from build123d import *

# Parameters (mm, degrees)
SALIENTE_EXTRUIR1_DEPTH = 4
SALIENTE_EXTRUIR2_DEPTH = 6.2
CORTAR_EXTRUIR1_REACH   = 20.8
CROQUIS3_R              = 1.6
CORTAR_EXTRUIR2_DEPTH   = 3
SALIENTE_EXTRUIR3_DEPTH = 8.4
SALIENTE_EXTRUIR4_DEPTH = 10


with BuildPart() as part:
    # Croquis1 → Saliente-Extruir1 (new body)
    with BuildSketch(Plane.XY):
        Polygon((0, 0), (25, 0), (25, 5), (13.5, 5), (13.5, 35), (0, 35), align=None)
    extrude(amount=SALIENTE_EXTRUIR1_DEPTH)

    # Croquis2 → Saliente-Extruir2 (add)
    with BuildSketch(Plane.XY.offset(4)):
        Polygon((6.2, 35), (6.2, 0), (25, 0), (25, 5), (13.5, 5), (13.5, 35), align=None)
    extrude(amount=SALIENTE_EXTRUIR2_DEPTH)

    # Croquis3 → Cortar-Extruir1 (cut, up to next)
    with BuildSketch(Plane.ZY.offset(-6.2), mode=Mode.PRIVATE) as cortar_extruir1_sk1:
        with Locations((7.1, 24.3)):
            Circle(CROQUIS3_R)
    cortar_extruir1_tool1 = extrude(cortar_extruir1_sk1.sketch, amount=-CORTAR_EXTRUIR1_REACH, mode=Mode.PRIVATE) & part.part
    add(cortar_extruir1_tool1.solids().sort_by_distance((6.2, 24.3, 7.1))[0], mode=Mode.SUBTRACT)

    # Croquis4 → Cortar-Extruir2 (cut)
    with BuildSketch(Plane(origin=(13.5, 0, 0), x_dir=(0, 0, -1), z_dir=(1, 0, 0))):
        Polygon((-7.1, 27.590896534), (-9.95, 25.945448267), (-9.95, 22.654551733), (-7.1, 21.009103466), (-4.25, 22.654551733), (-4.25, 25.945448267), align=None)
    extrude(amount=-CORTAR_EXTRUIR2_DEPTH, mode=Mode.SUBTRACT)

    # Croquis5 → Saliente-Extruir3 (add)
    with BuildSketch(Plane.XZ):
        Polygon((0, 0), (25, 0), (25, 10.2), (6.2, 10.2), (6.2, 4), (0, 4), align=None)
    extrude(amount=SALIENTE_EXTRUIR3_DEPTH)

    # Croquis6 → Saliente-Extruir4 (add)
    with BuildSketch(Plane.XZ.offset(8.4)):
        Polygon((17, 0), (17, 10.2), (6.2, 10.2), (6.2, 4), (0, 4), (0, 0), align=None)
    extrude(amount=SALIENTE_EXTRUIR4_DEPTH)


solid = part.part
CAD build for the part. Positions are in the model's coordinates, mm. A direction names the side the tool comes from. Coordinates: 2 decimals unless noted, no trailing zeros. Write each loop counter-clockwise with the first axis right and the second up, starting at its lowest first coordinate (ties: lowest second). Pieces come first, ordered by that corner, then holes. Notation, with made-up numbers: M -35.5,-4.5 L 0.5,-4.5 A31 ccw 0.5,26.5 Z; hole C 54.5,-34 d11. An arc over 180 degrees is marked long. Answer as a JSON object with one key per item and string values. Group by question number.
1) Saw through at A-A (y = 24.3). Write the cut outline in (x, z), plus the area to 3 significant figures.
2) Mould opens along Z. For faces 1 (the face through (12.02, 21.84, 8.54)), 2 (the face through (6.2, 9, 7)), 3 (the face through (3, 9, 4)) say: +Z half, -Z half, draft (parallel to the pull), parting line (faces both ways), or undercut.
3) Pin check, flat tips, straight feed: pin 1 Ø3 at (y, z) = (-9.5, 3) entering from -X; pin 2 Ø2 at (x, z) = (18.5, 1) entering from -Y; pin 3 Ø2.5 at (y, z) = (24.3, 7.1) entering from +X; pin 4 Ø3 at (x, y) = (3, 8.5) entering from +Z. Stop position of each tip, or through.
4) Saw through at C-C (y = -3). Write the cut outline in (x, z).
5) Tool access for faces 4 (the face through (21, -8.4, 5)), 5 (the face through (12, 24, 4.25)), 6 (the face through (13.5, 20, 5)): list every direction of +Z, -Z, +X, -X, +Y, -Y with a clear straight run to the whole face (end or side of a thin tool).
6) Wall check: line 1 (Y direction, x = 7.8, z = 7.1); line 2 (X direction, y = 25, z = 4.5); line 3 (Y direction, x = 19.75, z = 3). Give the ranges that are in metal, low to high. Write a range as from..to.
7) Saw through at D-D (x = 23). Write the cut outline in (y, z).
8) Saw through at B-B (z = 6.5). Write the cut outline in (x, y).
Values follow:
{
 "1": {"outline": "M 0,0 L 13.5,0 L 13.5,4.25 L 10.5,4.25 L 10.5,5.5 L 6.2,5.5 L 6.2,4 L 0,4 Z; M 6.2,8.7 L 10.5,8.7 L 10.5,9.95 L 13.5,9.95 L 13.5,10.2 L 6.2,10.2 Z", "area": "68.4 mm2"},
 "2": {"face 1": "undercut", "face 2": "draft", "face 3": "+Z half"},
 "3": {"pin 1": "stops at x = 0", "pin 2": "stops at y = -8.4", "pin 3": "passes through", "pin 4": "stops at z = 4"},
 "4": {"outline": "M 0,0 L 25,0 L 25,10.2 L 6.2,10.2 L 6.2,4 L 0,4 Z"},
 "5": {"face 4": "+Z, -Z, +X, -Y", "face 5": "+X", "face 6": "+Z, -Z, +X, +Y"},
 "6": {"line 1": "y = -18.4..22.7, 25.9..35", "line 2": "x = 6.2..10.5", "line 3": "y = -8.4..5"},
 "7": {"outline": "M -8.4,0 L 5,0 L 5,10.2 L -8.4,10.2 Z"},
 "8": {"outline": "M 6.2,-18.4 L 17,-18.4 L 17,-8.4 L 25,-8.4 L 25,5 L 13.5,5 L 13.5,21.36 L 10.5,21.36 L 10.5,22.82 L 6.2,22.82 Z; M 6.2,25.78 L 10.5,25.78 L 10.5,27.24 L 13.5,27.24 L 13.5,35 L 6.2,35 Z"}
}
